```python
from build123d import *

# Parameters (mm, degrees)
F0_W      = 6
F0_H      = 60
F1_DEPTH  = 2
F3_DEPTH  = 6
F6_DEPTH  = 25
F4_W      = 1
F4_H      = 20
F7_DEPTH  = 2
F9_DEPTH  = 10
F10_R     = 0.5
F11_DEPTH = 10


# Not quite as in the source:
# - a feature of the source that left no trace in its solid (it failed there, or was rolled back) is left out
# - the program builds the solid bodies; features that only make, move or delete a surface that nothing else refers to are left out


with BuildPart() as f1:
    # F0 (on Top) → F1 (new body)
    with BuildSketch(Plane.XY):
        Rectangle(F0_W, F0_H)
    extrude(amount=F1_DEPTH)

    # F2 (on face) → F3 (join)
    with BuildSketch(Plane.YZ.offset(3)):
        with BuildLine():
            Line((28, 6), (30, 6))
            ThreePointArc((30, 6), (26, 10), (22, 6))
            Line((22, 6), (24, 6))
            ThreePointArc((24, 6), (26, 8), (28, 6))
        make_face()
        with BuildLine():
            Line((22, 2), (30, 2))
            Line((30, 2), (30, 6))
            Line((30, 6), (28, 6))
            ThreePointArc((28, 6), (26, 4), (24, 6))
            Line((24, 6), (22, 6))
            Line((22, 6), (22, 2))
        make_face()
    extrude(amount=-F3_DEPTH)

    # F5 (on face) → F6 (cut)
    with BuildSketch(Plane.XY.offset(2)):
        Polygon((1.6, 22), (1.6, 30), (0, 30), (-1.6, 30), (-1.6, 22), align=None)
    extrude(amount=F6_DEPTH, mode=Mode.SUBTRACT)

    # F4 (on face) → F7 (join)
    with BuildSketch(Plane.XY.offset(2)):
        with Locations((2.5, -3.7680014595)):
            Rectangle(F4_W, F4_H)
        with Locations((-2.5, -3.7680014595)):
            Rectangle(F4_W, F4_H)
    extrude(amount=F7_DEPTH)

    # F8 (on face) → F9 (join)
    with BuildSketch(Plane.XZ.offset(13.7680014595)):
        with BuildLine():
            ThreePointArc((2.5, 3.5), (2.1464466094, 3.3535533906), (2, 3))
            ThreePointArc((2, 3), (2.5, 2.5), (3, 3))
            ThreePointArc((3, 3), (2.8535533906, 3.3535533906), (2.5, 3.5))
        make_face()
        with BuildLine():
            ThreePointArc((-2.5, 3.5), (-2.8535533906, 2.6464466094), (-2, 3))
            ThreePointArc((-2, 3), (-2.1464466094, 3.3535533906), (-2.5, 3.5))
        make_face()
    extrude(amount=F9_DEPTH)

    # F10 (on face) → F11 (join)
    with BuildSketch(Plane(origin=(0, 6.2319985405, 0), x_dir=(-1, 0, 0), z_dir=(0, 1, 0))):
        with Locations((-2.5, 3)):
            Circle(F10_R)
        with Locations((2.5, 3)):
            Circle(F10_R)
    extrude(amount=F11_DEPTH)


solid = f1.part
```
For this review, take the finished solid that the model builds, in its own axes (mm). A direction names the side the tool comes from. Round coordinates to 2 decimals unless told otherwise and drop trailing zeros. Write each loop counter-clockwise with the first axis right and the second up, starting at its lowest first coordinate (ties: lowest second). Pieces come first, ordered by that corner, then holes. Notation, with made-up numbers: M 79.5,75 L 94.5,75 A17 ccw 94.5,105 Z; hole C 32,5.5 d6. An arc over 180 degrees is marked long. One line per item, written item: value. Start each with the question number.
(1) The part is to be moulded in two halves that separate along X. For faces 1 (the cylindrical face through (3, 11, 3)), 2 (the cylindrical face through (2.31, 27.908, 5.399)), say which applies: released by +X, released by -X, zero draft, split by the parting line, or undercut.
(2) Machinability: for faces 3 (the flat face through (-2, -4, 3)), 4 (the flat face through (2.5, -23.768, 3)), 5 (the flat face through (-1.6, 25, 4)), 6 (the flat face through (2.5, 6.232, 3.7)), 7 (the cylindrical face through (-2, 11, 3)), which of the approach directions +Z, -Z, +X, -X, +Y, -Y give a long, thin tool a straight path to every point of the face, cutting with its end or side? Answer none if there is none.
(3) Wall thickness on line 1 (Y direction, x = -2.35, z = 6); line 2 (X direction, y = 23.5, z = 7.25); line 3 (Z direction, x = 2.7, y = 26): over which ranges is each line inside the solid? List them lowest first.
(4) Insertion check: pin 1 (0.8 mm diameter, centred on x = 2.5, z = 2.5, fed in from -Y); pin 2 (1.1 mm diameter, centred on x = -2, z = 4, fed in from -Y); pin 3 (3.5 mm diameter, centred on y = 26, z = 6, fed in from +X); pin 4 (0.8 mm diameter, centred on x = -2.5, y = -5.5, fed in from +Z). Each pin has a flat end and moves straight along its axis. Give the tip position at first contact, or say it passes through.
(5) We need section B-B (z = 5.25). Give the boundary of the cut face in (x, y), and give its area (3 significant figures).
(6) We need section A-A (y = -10.5). Give the boundary of the cut face in (x, z), and give its area (3 significant figures).
(7) We need section C-C (y = 8.5). Give the boundary of the cut face in (x, z), and give its area (3 significant figures).
Result:
1. face 1: undercut
1. face 2: zero draft
2. face 3: +Z, -Y
2. face 4: +Z, +X, -X, -Y
2. face 5: +Z, +Y, -Y
2. face 6: +Z
2. face 7: none
3. line 1: 22 to 24, 28 to 30
3. line 2: -3 to -1.6, 1.6 to 3
3. line 3: 0 to 4, 8 to 10
4. pin 1: y = -23.77
4. pin 2: y = -13.77
4. pin 3: through
4. pin 4: z = 4
5. outline: M -3,22 L -1.6,22 L -1.6,24.15 L -3,24.15 Z; M -3,27.85 L -1.6,27.85 L -1.6,30 L -3,30 Z; M 1.6,22 L 3,22 L 3,24.15 L 1.6,24.15 Z; M 1.6,27.85 L 3,27.85 L 3,30 L 1.6,30 Z
5. area: 12.0 mm²
6. outline: M -3,0 L 3,0 L 3,4 L 2,4 L 2,2 L -2,2 L -2,4 L -3,4 Z
6. area: 16.0 mm²
7. outline: M -3,0 L 3,0 L 3,2 L -3,2 Z; C -2.5,3 d1; C 2.5,3 d1
7. area: 13.6 mm²
